Geometry: final body of the model. Coordinates: model frame, mm. Round coordinates to 2 decimals unless told otherwise and drop trailing zeros. Loops run counter-clockwise (first coordinate to the right, second up) from the corner with the lowest first, then second, coordinate; pieces in that order, holes last. Notation, with made-up numbers: (-20, 14) - (11, 14) arc R27 ccw to (11, 53) - close; hole circle Ø5 at (-22.75, -34). An arc over 180 degrees is marked (long way). Use CSV: the item, a comma, the result in double quotes.
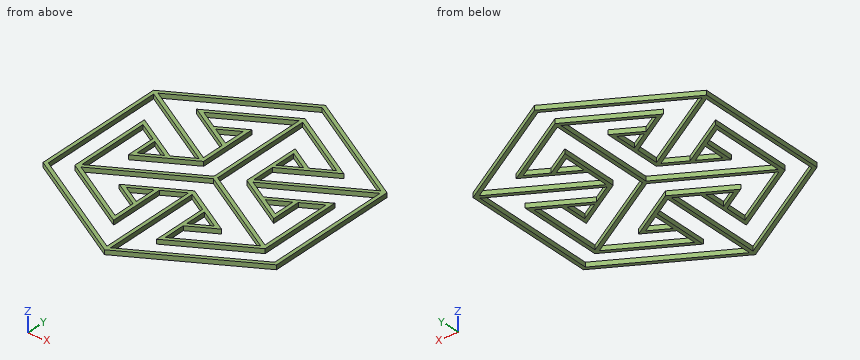
from build123d import *

# Parameters (mm, degrees)
F1_DEPTH = 2


with BuildPart() as f1:
    # F0 (on Top) → F1 (new body)
    with BuildSketch(Plane.XY):
        Polygon((0, 60), (-51.961524, 30), (-51.961524, -30), (0, -60), (51.961524, -30), (51.961524, 30), align=None)
        Polygon((-11.2, -19.398969), (-11.2, -29.054026), (-19.561524, -24.226497), align=None, mode=Mode.SUBTRACT)
        Polygon((-50.361524, -29.07624), (-50.361524, 28.152479), (-12, 6.004443), (-20.8, 0.92376), (-42.361524, 13.372312), (-42.361524, -24.457437), (-9.6, -43.372312), (-9.6, -18.475209), (-0.8, -13.394526), (-0.8, -57.690599), align=None, mode=Mode.SUBTRACT)
        Polygon((0, -11.085125), (-22.761524, -24.226497), (-11.2, -30.901546), (-11.2, -40.601031), (-39.961524, -23.995557), (0, -0.92376), (39.961524, -23.995557), (11.2, -40.601031), (11.2, -30.901546), (22.761524, -24.226497), align=None, mode=Mode.SUBTRACT)
        Polygon((11.2, -19.398969), (19.561524, -24.226497), (11.2, -29.054026), align=None, mode=Mode.SUBTRACT)
        Polygon((50.361524, -29.07624), (0.8, -57.690599), (0.8, -13.394526), (9.6, -18.475209), (9.6, -43.372312), (42.361524, -24.457437), (42.361524, 13.372312), (20.8, 0.92376), (12, 6.004443), (50.361524, 28.152479), align=None, mode=Mode.SUBTRACT)
        Polygon((-22.4, 0), (-30.761524, -4.827528), (-30.761524, 4.827528), align=None, mode=Mode.SUBTRACT)
        Polygon((-40.761524, -22.609917), (-40.761524, 10.601031), (-32.361524, 5.751289), (-32.361524, -7.59881), (-9.6, 5.542563), (-9.6, 31.825307), (-21.161524, 25.150258), (-29.561524, 30), (-0.8, 46.605474), (-0.8, 0.46188), align=None, mode=Mode.SUBTRACT)
        Polygon((-11.2, 29.054026), (-11.2, 19.398969), (-19.561524, 24.226497), align=None, mode=Mode.SUBTRACT)
        Polygon((0, 48.914875), (-32.761524, 30), (-11.2, 17.551448), (-11.2, 7.390083), (-49.561524, 29.53812), (0, 58.152479), (49.561524, 29.53812), (11.2, 7.390083), (11.2, 17.551448), (32.761524, 30), align=None, mode=Mode.SUBTRACT)
        Polygon((0.8, 46.605474), (29.561524, 30), (21.161524, 25.150258), (9.6, 31.825307), (9.6, 5.542563), (32.361524, -7.59881), (32.361524, 5.751289), (40.761524, 10.601031), (40.761524, -22.609917), (0.8, 0.46188), align=None, mode=Mode.SUBTRACT)
        Polygon((19.561524, 24.226497), (11.2, 19.398969), (11.2, 29.054026), align=None, mode=Mode.SUBTRACT)
        Polygon((30.761524, -4.827528), (22.4, 0), (30.761524, 4.827528), align=None, mode=Mode.SUBTRACT)
    extrude(amount=F1_DEPTH)


solid = f1.part
Item 1: Pin query (flat end, axial travel): P1, Ø1, axis at y = -42.5, z = 0.5, coming from the +X side; P2, Ø1, axis at y = -36.5, z = 1, coming from the +X side. Return the tip coordinate at first contact, or that it passes through.
Final values:
P1,"stops at x = 31.18"
P2,"stops at x = 41.57"
Item 2: Material intervals for line 1 (Y direction, x = 0, z = 1.8); line 2 (X direction, y = -48, z = 1.65); line 3 (Y direction, x = -9.5, z = 1.5), sorted ascending.
Final values:
line 1,"y = -60 to -11.09, -0.92 to 48.91, 58.15 to 60"
line 2,"x = -20.78 to -17.58, -0.8 to 0.8, 17.58 to 20.78"
line 3,"y = -54.52 to -52.67, -18.42 to -16.57, -6.41 to -4.56, 41.58 to 43.43, 52.67 to 54.52"
Item 3: Section D-D on y = -32.5. Return the cut outline in (x, z), plus the area to 3 significant figures.
Final values:
outline,"(-47.63, 0) - (-44.43, 0) - (-44.43, 2) - (-47.63, 2) - close; (-28.43, 0) - (-25.23, 0) - (-25.23, 2) - (-28.43, 2) - close; (-11.2, 0) - (-9.6, 0) - (-9.6, 2) - (-11.2, 2) - close; (-0.8, 0) - (0.8, 0) - (0.8, 2) - (-0.8, 2) - close; (9.6, 0) - (11.2, 0) - (11.2, 2) - (9.6, 2) - close; (25.23, 0) - (28.43, 0) - (28.43, 2) - (25.23, 2) - close; (44.43, 0) - (47.63, 0) - (47.63, 2) - (44.43, 2) - close"
area,"35.2 mm²"
Item 4: Section C-C on x = -4.5. Return the cut outline in (y, z).
Final values:
outline,"(-57.4, 0) - (-55.55, 0) - (-55.55, 2) - (-57.4, 2) - close; (-15.53, 0) - (-13.68, 0) - (-13.68, 2) - (-15.53, 2) - close; (-3.52, 0) - (-1.67, 0) - (-1.67, 2) - (-3.52, 2) - close; (44.47, 0) - (46.32, 0) - (46.32, 2) - (44.47, 2) - close; (55.55, 0) - (57.4, 0) - (57.4, 2) - (55.55, 2) - close"
Item 5: Section B-B on y = 34. Return the cut outline in (x, z).
Final values:
outline,"(-45.03, 0) - (-41.83, 0) - (-41.83, 2) - (-45.03, 2) - close; (-25.83, 0) - (-22.63, 0) - (-22.63, 2) - (-25.83, 2) - close; (-0.8, 0) - (0.8, 0) - (0.8, 2) - (-0.8, 2) - close; (22.63, 0) - (25.83, 0) - (25.83, 2) - (22.63, 2) - close; (41.83, 0) - (45.03, 0) - (45.03, 2) - (41.83, 2) - close"
Item 6: Section A-A on x = -44.5. Return the cut outline in (y, z).
Final values:
outline,"(-34.31, 0) - (-32.46, 0) - (-32.46, 2) - (-34.31, 2) - close; (24.77, 0) - (26.62, 0) - (26.62, 2) - (24.77, 2) - close; (32.46, 0) - (34.31, 0) - (34.31, 2) - (32.46, 2) - close"
